Geometry check sheet. Reference: the model listing, model coordinates, mm. Face numbers are marked on the shaded views. Round coordinates to 2 decimals unless told otherwise and drop trailing zeros. Loops run counter-clockwise (first coordinate to the right, second up) from the corner with the lowest first, then second, coordinate; pieces in that order, holes last. Notation, with made-up numbers: M 16,11 L 32,11 A24 ccw 32,48 Z; hole C 30.25,48 d6. An arc over 180 degrees is marked long. Use one line per item in the form item = value. Start each with the question number.
1. Go/stop test with flat-tipped pins: pin 1 (4 mm diameter, centred on x = -21.5, y = 13, fed in from +Z); pin 2 (7 mm diameter, centred on x = -35.5, y = 5.5, fed in from +Z). Record where each tip stops, or that it passes through.
2. Cross-section at B-B (y = 35.5). Record the boundary of the cut face in (x, z).
3. Material ranges on line 1 (Y direction, x = -5.5, z = 1.45); line 2 (Z direction, x = -15, y = 26.5); line 3 (X direction, y = 18, z = 4.4), recorded low to high.
4. Cross-section at C-C (x = -35.5). Record the boundary of the cut face in (y, z), then the cut area to 3 significant figures.
5. Cross-section at D-D (y = 9.5). Record the boundary of the cut face in (x, z).
6. Cross-section at A-A (z = 3.1). Record the boundary of the cut face in (x, y).
7. Draft check along X on the marked faces 1, 2, 3 and 4. Enter one of: pulls with the +X half, pulls with the -X half, needs draft (parallel to the pull), parting line crosses it, or undercut.
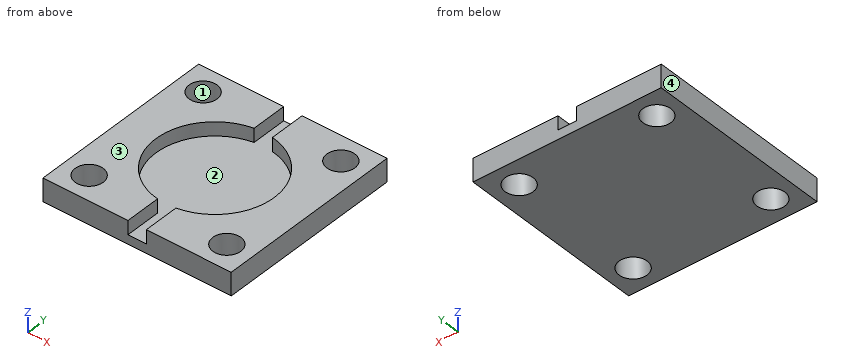
```python
from build123d import *

# Parameters (mm, degrees)
CROQUIS1_W             = 41
CROQUIS1_H             = 41
PLAQUEBASE_DEPTH       = 5
CROQUIS2_R             = 12.86
CERCLECENTRAL_DEPTH    = 3
CROQUIS3_R             = 3.05
SUPPORT_DEPTH          = 5
CROQUIS4_W             = 3
CROQUIS4_H             = 2.5
TROUSLAT_DEPTH         = 41
CORTAR_EXTRUIR1_DEPTH  = 0.5
CORTAR_EXTRUIR2_DEPTH  = 0.5
CROQUIS15_W            = 7.727780146
CROQUIS15_H            = 3
CORTAR_EXTRUIR3_DEPTH  = 0.5
CROQUIS16_W            = 7.727780146
CROQUIS16_H            = 3
CORTAR_EXTRUIR4_DEPTH  = 0.5
CROQUIS17_W            = 7.727780146
CROQUIS17_H            = 3
CORTAR_EXTRUIR5_DEPTH  = 0.5
CROQUIS18_W            = 7.727780146
CROQUIS18_H            = 3
CORTAR_EXTRUIR6_DEPTH  = 0.5
CROQUIS19_W            = 0.5
CROQUIS19_H            = 3
CORTAR_EXTRUIR7_DEPTH  = 0.5
CROQUIS20_W            = 0.5
CROQUIS20_H            = 3
CORTAR_EXTRUIR8_DEPTH  = 0.5
CROQUIS21_W            = 0.5
CROQUIS21_H            = 3
CORTAR_EXTRUIR9_DEPTH  = 0.5
CROQUIS22_W            = 0.5
CROQUIS22_H            = 3
CORTAR_EXTRUIR10_DEPTH = 0.5


with BuildPart() as part:
    # Croquis1 → PlaqueBase (new body)
    with BuildSketch(Plane(origin=(0, 0, 0), x_dir=(0, 1, 0), z_dir=(0, 0, 1))):
        with Locations((20.5, 20.5)):
            Rectangle(CROQUIS1_W, CROQUIS1_H)
    extrude(amount=PLAQUEBASE_DEPTH)

    # Croquis2 → CercleCentral (cut)
    with BuildSketch(Plane.XY.offset(5)):
        with Locations((-20.5, 20.5)):
            Circle(CROQUIS2_R)
    extrude(amount=-CERCLECENTRAL_DEPTH, mode=Mode.SUBTRACT)

    # Croquis3 → Support (cut)
    with BuildSketch(Plane.XY.offset(5)):
        with Locations((-35.5, 5.5)):
            Circle(CROQUIS3_R)
        with Locations((-5.5, 5.5)):
            Circle(CROQUIS3_R)
        with Locations((-5.5, 35.5)):
            Circle(CROQUIS3_R)
        with Locations((-35.5, 35.5)):
            Circle(CROQUIS3_R)
    extrude(amount=-SUPPORT_DEPTH, mode=Mode.SUBTRACT)

    # Croquis4 → TrousLat (cut)
    with BuildSketch(Plane(origin=(0, 0, 0), x_dir=(-1, 0, 0), z_dir=(0, -1, 0))):
        with Locations((20.5, -3.75)):
            Rectangle(CROQUIS4_W, CROQUIS4_H)
    extrude(amount=-TROUSLAT_DEPTH, mode=Mode.SUBTRACT)

    # Croquis6 → Cortar-Extruir1 (cut)
    with BuildSketch(Plane.XY.offset(2.5)):
        with BuildLine():
            Line((-19, 33.272219854), (-19, 41))
            Line((-19, 41), (-22, 41))
            Line((-22, 41), (-22, 33.272219854))
            ThreePointArc((-22, 33.272219854), (-20.5, 33.36), (-19, 33.272219854))
        make_face()
    extrude(amount=-CORTAR_EXTRUIR1_DEPTH, mode=Mode.SUBTRACT)

    # Croquis14 → Cortar-Extruir2 (cut)
    with BuildSketch(Plane.XY.offset(2.5)):
        with BuildLine():
            Line((-22, 7.727780146), (-22, 0))
            Line((-22, 0), (-19, 0))
            Line((-19, 0), (-19, 7.727780146))
            ThreePointArc((-19, 7.727780146), (-20.5, 7.64), (-22, 7.727780146))
        make_face()
    extrude(amount=-CORTAR_EXTRUIR2_DEPTH, mode=Mode.SUBTRACT)

    # Croquis15 → Cortar-Extruir3 (cut)
    with BuildSketch(Plane(origin=(-19, 0, 0), x_dir=(0, -1, 0), z_dir=(-1, 0, 0))):
        with Locations((-37.136109927, 3.5)):
            Rectangle(CROQUIS15_W, CROQUIS15_H)
    extrude(amount=-CORTAR_EXTRUIR3_DEPTH, mode=Mode.SUBTRACT)

    # Croquis16 → Cortar-Extruir4 (cut)
    with BuildSketch(Plane(origin=(-19, 0, 0), x_dir=(0, -1, 0), z_dir=(-1, 0, 0))):
        with Locations((-3.863890073, 3.5)):
            Rectangle(CROQUIS16_W, CROQUIS16_H)
    extrude(amount=-CORTAR_EXTRUIR4_DEPTH, mode=Mode.SUBTRACT)

    # Croquis17 → Cortar-Extruir5 (cut)
    with BuildSketch(Plane.YZ.offset(-22)):
        with Locations((3.863890073, 3.5)):
            Rectangle(CROQUIS17_W, CROQUIS17_H)
    extrude(amount=-CORTAR_EXTRUIR5_DEPTH, mode=Mode.SUBTRACT)

    # Croquis18 → Cortar-Extruir6 (cut)
    with BuildSketch(Plane.YZ.offset(-22)):
        with Locations((37.136109927, 3.5)):
            Rectangle(CROQUIS18_W, CROQUIS18_H)
    extrude(amount=-CORTAR_EXTRUIR6_DEPTH, mode=Mode.SUBTRACT)

    # Croquis19 → Cortar-Extruir7 (cut)
    with BuildSketch(Plane.XZ.offset(-7.727780146)):
        with Locations((-22.25, 3.5)):
            Rectangle(CROQUIS19_W, CROQUIS19_H)
    extrude(amount=-CORTAR_EXTRUIR7_DEPTH, mode=Mode.SUBTRACT)

    # Croquis20 → Cortar-Extruir8 (cut)
    with BuildSketch(Plane.XZ.offset(-7.727780146)):
        with Locations((-18.75, 3.5)):
            Rectangle(CROQUIS20_W, CROQUIS20_H)
    extrude(amount=-CORTAR_EXTRUIR8_DEPTH, mode=Mode.SUBTRACT)

    # Croquis21 → Cortar-Extruir9 (cut)
    with BuildSketch(Plane(origin=(0, 33.272219854, 0), x_dir=(-1, 0, 0), z_dir=(0, 1, 0))):
        with Locations((18.75, 3.5)):
            Rectangle(CROQUIS21_W, CROQUIS21_H)
    extrude(amount=-CORTAR_EXTRUIR9_DEPTH, mode=Mode.SUBTRACT)

    # Croquis22 → Cortar-Extruir10 (cut)
    with BuildSketch(Plane(origin=(0, 33.272219854, 0), x_dir=(-1, 0, 0), z_dir=(0, 1, 0))):
        with Locations((22.25, 3.5)):
            Rectangle(CROQUIS22_W, CROQUIS22_H)
    extrude(amount=-CORTAR_EXTRUIR10_DEPTH, mode=Mode.SUBTRACT)


solid = part.part
```
Reported:
q1.pin_1 = 2
q1.pin_2 = 5
q2.outline = M -41,0 L -38.55,0 L -38.55,5 L -41,5 Z; M -32.45,0 L -8.55,0 L -8.55,5 L -18.5,5 L -18.5,2 L -22.5,2 L -22.5,5 L -32.45,5 Z; M -2.45,0 L 0,0 L 0,5 L -2.45,5 Z
q3.line_1 = 0 to 2.45, 8.55 to 32.45, 38.55 to 41
q3.line_2 = 0 to 2
q3.line_3 = -41 to -33.11, -7.89 to 0
q4.outline = M 0,0 L 2.45,0 L 2.45,5 L 0,5 Z; M 8.55,0 L 32.45,0 L 32.45,5 L 8.55,5 Z; M 38.55,0 L 41,0 L 41,5 L 38.55,5 Z
q4.area = 144 mm²
q5.outline = M -41,0 L 0,0 L 0,5 L -13.84,5 L -13.84,2 L -27.16,2 L -27.16,5 L -41,5 Z
q6.outline = M -41,0 L -22.5,0 L -22.5,7.8 A12.86 cw -22.5,33.2 L -22.5,41 L -41,41 Z; M -18.5,0 L 0,0 L 0,41 L -18.5,41 L -18.5,33.2 A12.86 cw -18.5,7.8 Z; hole C -35.5,5.5 d6.1; hole C -35.5,35.5 d6.1; hole C -5.5,5.5 d6.1; hole C -5.5,35.5 d6.1
q7.face_1 = undercut
q7.face_2 = undercut
q7.face_3 = needs draft
q7.face_4 = pulls with the -X half
